The figure shows three views and two pictorial views of one solid part (mm, origin at its lowest corner). Answer the questions. A direction names the side the tool comes from. Give positions to 0.01 mm unless a question says otherwise; leave off trailing zeros. Loops run counter-clockwise (first coordinate to the right, second up) from the corner with the lowest first, then second, coordinate; pieces in that order, holes last. Notation, with made-up numbers: (10.25, -8.75) - (39.25, -8.75) arc R28 ccw to (39.25, 29.25) - close; hole circle Ø11 at (0.25, 36). An arc over 180 degrees is marked (long way). One line per question, with ' | ' between items.
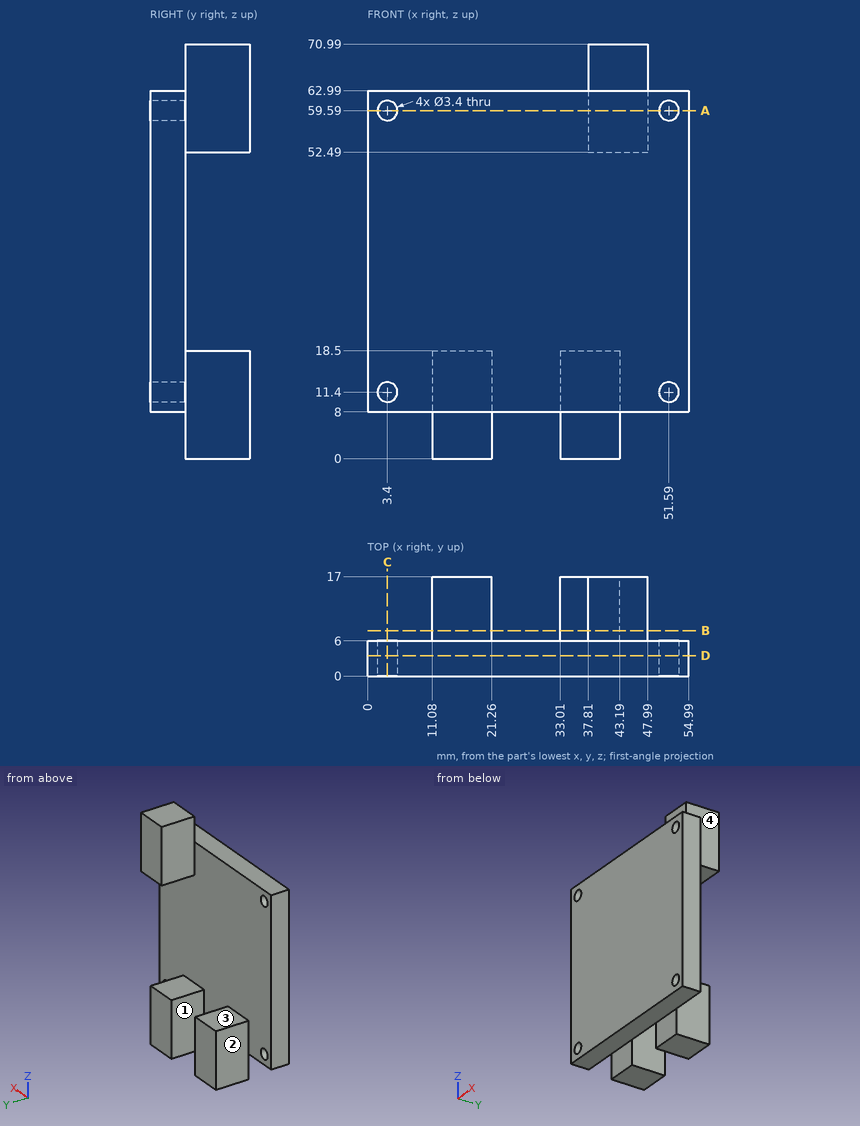
1. Find section A-A on z = 59.59. Write down the section's boundary in (x, y).
Evaluation:
outline: (0, 0) - (1.7, 0) - (1.7, 6) - (0, 6) - close; (5.1, 0) - (49.89, 0) - (49.89, 6) - (47.99, 6) - (47.99, 17) - (37.81, 17) - (37.81, 6) - (5.1, 6) - close; (53.29, 0) - (54.99, 0) - (54.99, 6) - (53.29, 6) - close
2. Which of the six approach directions +Z, -Z, +X, -X, +Y, -Y give full straight-line access (tool end or side, diameter ignored) to the marked faces 1, 2, 3 and 4?
Evaluation:
face 1: +Z, -Z, +Y | face 2: +Z, -Z, -X, +Y | face 3: +Z, +X, -X, +Y | face 4: +Z, -Z, +X, +Y
3. Find section D-D on y = 3.5. Write down the section's boundary in (x, z).
Evaluation:
outline: (0, 8) - (54.99, 8) - (54.99, 62.99) - (0, 62.99) - close; hole circle Ø3.4 at (3.4, 11.4); hole circle Ø3.4 at (3.4, 59.59); hole circle Ø3.4 at (51.59, 11.4); hole circle Ø3.4 at (51.59, 59.59)
4. Find section C-C on x = 3.4. Write down the section's boundary in (y, z), then the cut area to 3 significant figures.
Evaluation:
outline: (0, 8) - (6, 8) - (6, 9.7) - (0, 9.7) - close; (0, 13.1) - (6, 13.1) - (6, 57.89) - (0, 57.89) - close; (0, 61.29) - (6, 61.29) - (6, 62.99) - (0, 62.99) - close | area: 289 mm2
5. Flat-ended cylindrical pins translate along their axes: pin 1 (8 mm diameter, centred on x = 43, y = 15, fed in from -Z); pin 2 (4 mm diameter, centred on x = 21.5, z = 59, fed in from +Y); pin 3 (2.5 mm diameter, centred on x = 3.4, z = 11.4, fed in from -Y); pin 4 (5 mm diameter, centred on x = 40.5, y = 2, fed in from -Z). Find the tip coordinate at first contact, or state that the pin passes through.
Evaluation:
pin 1: z = 0 | pin 2: y = 6 | pin 3: through | pin 4: z = 8
6. Find section B-B on y = 7.75. Write down the section's boundary in (x, z), then the cut area to 3 significant figures.
Evaluation:
outline: (11.08, 0) - (21.26, 0) - (21.26, 18.5) - (11.08, 18.5) - close; (33.01, 0) - (43.19, 0) - (43.19, 18.5) - (33.01, 18.5) - close; (37.81, 52.49) - (47.99, 52.49) - (47.99, 70.99) - (37.81, 70.99) - close | area: 565 mm2
7. Consider L1, parallel to X at y = 4.3, z = 59.59; L2, parallel to Z at x = 3.4, y = 3.4; L3, parallel to Z at x = 41.5, y = 12.25. Determine where each line is inside the solid, lowest interval first.
Evaluation:
L1: 0 to 1.7, 5.1 to 49.89, 53.29 to 54.99 | L2: 8 to 9.7, 13.1 to 57.89, 61.29 to 62.99 | L3: 0 to 18.5, 52.49 to 70.99
